CAD build for the part. Positions are in the model's coordinates, mm. Face numbers are marked on the shaded views. A direction names the side the tool comes from. Round coordinates to 2 decimals unless told otherwise and drop trailing zeros. Loops run counter-clockwise (first coordinate to the right, second up) from the corner with the lowest first, then second, coordinate; pieces in that order, holes last. Notation, with made-up numbers: (-34, 29.25) - (23, 29.25) arc R23 ccw to (23, 55.25) - close; hole circle Ø5 at (-37, 12.25). An arc over 180 degrees is marked (long way). Use one line per item in the form item = value.
from build123d import *

# Parameters (mm, degrees)
EXTRUDE001_DEPTH = 0.5
PAD001_DEPTH     = 3
SKETCH_W         = 45
SKETCH_H         = 20
SKETCH_R         = 4.25
PAD_DEPTH        = 24
SKETCH001_R      = 3.25
POCKET_DEPTH     = 20.001
SKETCH003_R      = 4.25
POCKET001_DEPTH  = 18
SKETCH004_R      = 1.65
POCKET002_DEPTH  = 7.75
FILLET_R         = 1.9


with BuildPart() as obj1:
    # path2990 → Extrude001 (new body)
    with BuildSketch(Plane(origin=(45, 9.801935, 12.357409), x_dir=(0, -1, 0), z_dir=(1, 0, 0))):
        with BuildLine():
            add(Edge.make_bspline(
                [(4.49398, 2.770757), (-4.49398, 2.770757)],
                knots=[0, 0, 28.94756, 28.94756], degree=1))
            add(Edge.make_bspline(
                [(-4.49398, 2.770757), (-4.49398, -2.598535)],
                knots=[0, 0, 20.9307, 20.9307], degree=1))
            add(Edge.make_bspline(
                [(-4.49398, -2.598535), (-3.433327, -2.598535)],
                knots=[0, 0, 3.41605, 3.41605], degree=1))
            add(Edge.make_bspline(
                [(-3.433327, -2.598535), (-3.433327, 1.788076)],
                knots=[0, 0, 17.09999, 17.09999], degree=1))
            add(Edge.make_bspline(
                [(-3.433327, 1.788076), (-0.680535, 1.788076)],
                knots=[0, 0, 8.86593, 8.86593], degree=1))
            add(Edge.make_bspline(
                [(-0.680535, 1.788076), (-0.680535, -2.319939)],
                knots=[0, 0, 16.01396, 16.01396], degree=1))
            add(Edge.make_bspline(
                [(-0.680535, -2.319939), (0.373986, -2.319939)],
                knots=[0, 0, 3.3963, 3.3963], degree=1))
            add(Edge.make_bspline(
                [(0.373986, -2.319939), (0.373986, 1.788076)],
                knots=[0, 0, 16.01396, 16.01396], degree=1))
            add(Edge.make_bspline(
                [(0.373986, 1.788076), (3.433327, 1.788076)],
                knots=[0, 0, 9.85323, 9.85323], degree=1))
            add(Edge.make_bspline(
                [(3.433327, 1.788076), (3.433327, -2.770757)],
                knots=[0, 0, 17.77135, 17.77135], degree=1))
            add(Edge.make_bspline(
                [(3.433327, -2.770757), (4.49398, -2.770757)],
                knots=[0, 0, 3.41605, 3.41605], degree=1))
            add(Edge.make_bspline(
                [(4.49398, -2.770757), (4.49398, 2.770757)],
                knots=[0, 0, 21.60206, 21.60206], degree=1))
        make_face()
    extrude(amount=-EXTRUDE001_DEPTH)


with BuildPart() as obj2:
    # Sketch005 → Pad001 (new body)
    with BuildSketch(Plane(origin=(22.5, 13.5, 5), x_dir=(1, 0, 0), z_dir=(0, 0, -1))):
        Polygon((-2.95, 14.703183), (-2.95, 1.703183), (0, 0), (2.95, 1.703183), (2.95, 14.703183), align=None)
    extrude(amount=PAD001_DEPTH)


with BuildPart() as obj3:
    # Sketch → Pad (new body)
    with BuildSketch(Plane.XY):
        with Locations((22.5, 10)):
            Rectangle(SKETCH_W, SKETCH_H)
        with Locations((10, 10)):
            Circle(SKETCH_R, mode=Mode.SUBTRACT)
        with Locations((35, 10)):
            Circle(SKETCH_R, mode=Mode.SUBTRACT)
    extrude(amount=PAD_DEPTH)

    # Sketch001 → Pocket (cut, through all)
    with BuildSketch(Plane.XZ):
        with Locations((22.5, 12)):
            Circle(SKETCH001_R)
    extrude(amount=-POCKET_DEPTH, mode=Mode.SUBTRACT)

    # Sketch003 → Pocket001 (cut)
    with BuildSketch(Plane(origin=(0, 20, 0), x_dir=(-1, 0, 0), z_dir=(0, 1, 0))):
        with Locations((-22.5, 12)):
            Circle(SKETCH003_R)
    extrude(amount=-POCKET001_DEPTH, mode=Mode.SUBTRACT)

    # Sketch004 → Pocket002 (cut)
    with BuildSketch(Plane(origin=(0, 0, 0), x_dir=(1, 0, 0), z_dir=(0, 0, -1))):
        with Locations((22.5, -10)):
            Circle(SKETCH004_R)
    extrude(amount=-POCKET002_DEPTH, mode=Mode.SUBTRACT)

    # Cut: cut obj2
    add(obj2.part, mode=Mode.SUBTRACT)

    # Cut001: cut obj1
    add(obj1.part, mode=Mode.SUBTRACT)

    # Fillet
    fillet_edges = [obj3.edges().sort_by_distance(p)[0] for p in [
        (45, 20, 12),
        (22.5, 20, 0),
        (22.5, 20, 24),
        (0, 20, 12),
        (45, 10, 0),
        (45, 10, 24),
        (45, 0, 12),
        (0, 10, 0),
        (22.5, 0, 0),
        (0, 10, 24),
        (22.5, 0, 24),
        (0, 0, 12),
    ]]
    fillet(fillet_edges, radius=FILLET_R)


solid = obj3.part
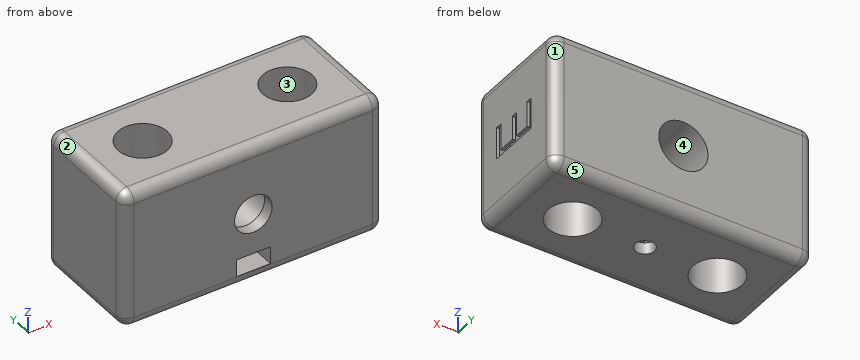
1) Two-plate mould, pull along Y, no slides. Class the marked faces 1, 2 and 3: +Y half, -Y half, draft (parallel to the pull), parting line (faces both ways), or undercut.
Report:
face_1 = +Y half
face_2 = draft
face_3 = undercut
2) Slice it at A-A (y = 17.25). Write the cut outline in (x, z), plus the area to 3 significant figures.
Report:
outline = (0, 1.9) arc R1.9 ccw to (1.9, 0) - (43.1, 0) arc R1.9 ccw to (45, 1.9) - (45, 22.1) arc R1.9 ccw to (43.1, 24) - (1.9, 24) arc R1.9 ccw to (0, 22.1) - close; hole circle Ø8.5 at (22.5, 12)
area = 1,020 mm^2
3) Tool access for the marked faces 4 and 5: list every direction of +Z, -Z, +X, -X, +Y, -Y with a clear straight run to the whole face (end or side of a thin tool).
Report:
face_4 = +Y
face_5 = -Z, +X, -X, +Y
4) Slice it at B-B (x = 35). Write the cut outline in (y, z), plus the area to 3 significant figures.
Report:
outline = (0, 1.9) arc R1.9 ccw to (1.9, 0) - (5.75, 0) - (5.75, 24) - (1.9, 24) arc R1.9 ccw to (0, 22.1) - close; (14.25, 0) - (18.1, 0) arc R1.9 ccw to (20, 1.9) - (20, 22.1) arc R1.9 ccw to (18.1, 24) - (14.25, 24) - close
area = 273 mm^2
5) Slice it at D-D (z = 4). Write the cut outline in (x, y), plus the area to 3 significant figures.
Report:
outline = (0, 1.9) arc R1.9 ccw to (1.9, 0) - (19.55, 0) - (19.55, 11.8) - (22.5, 13.5) - (25.45, 11.8) - (25.45, 0) - (43.1, 0) arc R1.9 ccw to (45, 1.9) - (45, 18.1) arc R1.9 ccw to (43.1, 20) - (1.9, 20) arc R1.9 ccw to (0, 18.1) - close; hole circle Ø8.5 at (10, 10); hole circle Ø8.5 at (35, 10)
area = 709 mm^2
6) Flat gauge pin, fed straight in: pin 1 (2.5 mm diameter, centred on x = 22.5, y = 10, fed in from -Z). Where does the tip first touch, or does it go through?
Report:
pin_1 = 7.75
7) Drill centre lines: probe 1 along X at (y, z) = (13.75, 4.5); probe 2 along Y at (x, z) = (35, 16); probe 3 along Y at (x, z) = (22.5, 5.7). Where is each one in solid material? Low to high.
Report:
probe_1 = 0 to 8, 12 to 33, 37 to 45
probe_2 = 0 to 5.75, 14.25 to 20
probe_3 = 0 to 8.35, 11.65 to 20
